```python
from build123d import *

# Parameters (mm, degrees)
F0_W     = 2.971
F0_H     = 2.971
F1_DEPTH = 4


with BuildPart() as f1:
    # F0 (on Top) → F1 (new body)
    with BuildSketch(Plane.XY):
        Polygon((-20.2072594216, -35), (20.2072594216, -35), (40.4145188433, 0), (20.2072594216, 35), (-20.2072594216, 35), (-40.4145188433, 0), align=None)
        with BuildLine():
            Line((21, -20), (-21, -20))
            ThreePointArc((-21, -20), (-23.5606601718, -21.0606601718), (-22.5, -18.5))
            Line((-22.5, -18.5), (-22.5, 18.5))
            ThreePointArc((-22.5, 18.5), (-23.5606601718, 21.0606601718), (-21, 20))
            Line((-21, 20), (21, 20))
            ThreePointArc((21, 20), (22.5, 21.5), (24, 20))
            ThreePointArc((24, 20), (23.5606601718, 18.9393398282), (22.5, 18.5))
            Line((22.5, 18.5), (22.5, -18.5))
            ThreePointArc((22.5, -18.5), (23.5606601718, -18.9393398282), (24, -20))
            ThreePointArc((24, -20), (22.5, -21.5), (21, -20))
        make_face(mode=Mode.SUBTRACT)
        with BuildLine():
            ThreePointArc((-22.5, -18.5), (-21.4393398282, -18.9393398282), (-21, -20))
            Line((-21, -20), (21, -20))
            ThreePointArc((21, -20), (21.4393398282, -18.9393398282), (22.5, -18.5))
            Line((22.5, -18.5), (22.5, 18.5))
            ThreePointArc((22.5, 18.5), (21.4393398282, 18.9393398282), (21, 20))
            Line((21, 20), (-21, 20))
            ThreePointArc((-21, 20), (-21.4393398282, 18.9393398282), (-22.5, 18.5))
            Line((-22.5, 18.5), (-22.5, -18.5))
        make_face()
        with BuildLine():
            Line((15.51465, -1.4855), (9.4855, -1.4855))
            Line((9.4855, -1.4855), (1.4855, -1.4855))
            Line((1.4855, -1.4855), (1.4855, -9.4855))
            Line((1.4855, -9.4855), (1.4855, -15.51465))
            ThreePointArc((1.4855, -15.51465), (0, -17.00015), (-1.4855, -15.51465))
            Line((-1.4855, -15.51465), (-1.4855, -9.4855))
            Line((-1.4855, -9.4855), (-1.4855, -1.4855))
            Line((-1.4855, -1.4855), (-9.4855, -1.4855))
            Line((-9.4855, -1.4855), (-15.51465, -1.4855))
            ThreePointArc((-15.51465, -1.4855), (-17.00015, 0), (-15.51465, 1.4855))
            Line((-15.51465, 1.4855), (-9.4855, 1.4855))
            Line((-9.4855, 1.4855), (-1.4855, 1.4855))
            Line((-1.4855, 1.4855), (-1.4855, 9.4855))
            Line((-1.4855, 9.4855), (-1.4855, 15.51465))
            ThreePointArc((-1.4855, 15.51465), (0, 17.00015), (1.4855, 15.51465))
            Line((1.4855, 15.51465), (1.4855, 9.4855))
            Line((1.4855, 9.4855), (1.4855, 1.4855))
            Line((1.4855, 1.4855), (9.4855, 1.4855))
            Line((9.4855, 1.4855), (15.51465, 1.4855))
            ThreePointArc((15.51465, 1.4855), (16.5650571235, 1.0504071235), (17.00015, 0))
            ThreePointArc((17.00015, 0), (16.5650571235, -1.0504071235), (15.51465, -1.4855))
        make_face(mode=Mode.SUBTRACT)
        with BuildLine():
            Line((-1.4855, 1.4855), (1.4855, 1.4855))
            Line((1.4855, 1.4855), (1.4855, 9.4855))
            ThreePointArc((1.4855, 9.4855), (0, 8), (-1.4855, 9.4855))
            Line((-1.4855, 9.4855), (-1.4855, 1.4855))
        make_face()
        with BuildLine():
            Line((-9.4855, -1.4855), (-1.4855, -1.4855))
            Line((-1.4855, -1.4855), (-1.4855, 1.4855))
            Line((-1.4855, 1.4855), (-9.4855, 1.4855))
            ThreePointArc((-9.4855, 1.4855), (-8.4350928765, 1.0504071235), (-8, 0))
            ThreePointArc((-8, 0), (-8.4350928765, -1.0504071235), (-9.4855, -1.4855))
        make_face()
        with BuildLine():
            Line((1.4855, -1.4855), (9.4855, -1.4855))
            ThreePointArc((9.4855, -1.4855), (8, 0), (9.4855, 1.4855))
            Line((9.4855, 1.4855), (1.4855, 1.4855))
            Line((1.4855, 1.4855), (1.4855, -1.4855))
        make_face()
        Rectangle(F0_W, F0_H)
        with BuildLine():
            Line((1.4855, -9.4855), (1.4855, -1.4855))
            Line((1.4855, -1.4855), (-1.4855, -1.4855))
            Line((-1.4855, -1.4855), (-1.4855, -9.4855))
            ThreePointArc((-1.4855, -9.4855), (0, -8), (1.4855, -9.4855))
        make_face()
    extrude(amount=F1_DEPTH)


solid = f1.part
```
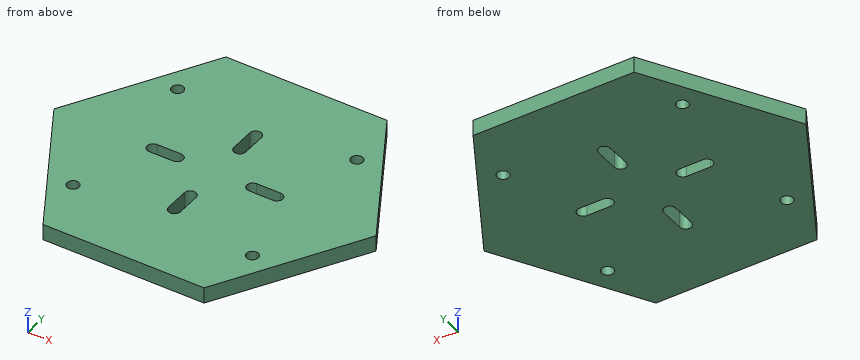
Input: part model. Units: mm. Frame: model coordinates. Round coordinates to 2 decimals unless told otherwise and drop trailing zeros. Write each loop counter-clockwise with the first axis right and the second up, starting at its lowest first coordinate (ties: lowest second). Pieces come first, ordered by that corner, then holes. Notation, with made-up numbers: M 21.25,45 L 45.25,45 A26 ccw 45.25,72 Z; hole C -8,89 d3. An arc over 180 degrees is marked long. Write each question's results on one line, items separated by ' | '.
Q1. Section query C-C (x = 0). Return loops of the section in (y, z), and give its area (3 significant figures).
Results:
outline: M -35,0 L -17,0 L -17,4 L -35,4 Z; M -8,0 L 8,0 L 8,4 L -8,4 Z; M 17,0 L 35,0 L 35,4 L 17,4 Z | area: 208 mm^2
Q2. Section query A-A (x = -14). Return loops of the section in (y, z), and give its area (3 significant figures).
Results:
outline: M -35,0 L -1.49,0 L -1.49,4 L -35,4 Z; M 1.49,0 L 35,0 L 35,4 L 1.49,4 Z | area: 268 mm^2
Q3. Pin query (flat end, axial travel): P1, Ø2.5, axis at x = -22.5, y = -20, coming from the +Z side; P2, Ø2, axis at y = -12.5, z = 1, coming from the -X side (3 decimals); P3, Ø1.5, axis at y = -1.5, z = 2.5, coming from the +X side; P4, Ø1.5, axis at x = 26.5, z = 2.5, coming from the +Y side. Return the tip coordinate at first contact, or that it passes through.
Results:
P1: passes through | P2: stops at x = -33.775 | P3: stops at x = 39.98 | P4: stops at y = 25.4
Q4. Section query B-B (z = 3.25). State how many separate pieces and enclosed holes the cut face has, and give its area (3 significant figures).
Results:
separate pieces: 1 | enclosed holes: 8 | area: 4,120 mm^2
Q5. Section query D-D (y = 27.5). Return loops of the section in (x, z), and give its area (3 significant figures).
Results:
outline: M -24.54,0 L 24.54,0 L 24.54,4 L -24.54,4 Z | area: 196 mm^2
Q6. Line query: line 1 along Y through (x, z) = (-11.5, 2.1); line 2 along X through (y, z) = (20, 1.9); line 3 along Y through (x, z) = (-22.5, 1.1). Output: solid intervals per line, ascending.
Results:
line 1: y = -35 to -1.49, 1.49 to 35 | line 2: x = -28.87 to -24, -21 to 21, 24 to 28.87 | line 3: y = -31.03 to -21.5, -18.5 to 18.5, 21.5 to 31.03
